from build123d import *

# Parameters (mm, degrees)
EXTRUDE_1_DEPTH     = 12
SKETCH_4_W          = 56
SKETCH_4_H          = 3
SKETCH_4_H_2        = 1
EXTRUDE_2_DEPTH     = 12
SKETCH_5_R          = 1.15
SKETCH_5_R_2        = 2.6
CUT_EXTRUDE_2_DEPTH = 53.211370172
SKETCH_7_R          = 1
CUT_EXTRUDE_3_DEPTH = 10


with BuildPart() as part:
    # 草图2 → 凸台-拉伸1 (new body)
    with BuildSketch(Plane(origin=(0, 0, 0), x_dir=(1, 0, 0), z_dir=(0, 1, 0))):
        Polygon((-10.725663717, 9.92920354), (45.274336283, 9.92920354), (45.274336283, -22.07079646), (-10.725663717, -22.07079646), (-10.725663717, -7.07079646), (-10.725663717, 1.92920354), align=None)
        Polygon((-9.725663717, -7.07079646), (-9.725663717, -14.07079646), (44.274336283, -14.07079646), (44.274336283, 8.92920354), (-9.725663717, 8.92920354), (-9.725663717, 0.92920354), align=None, mode=Mode.SUBTRACT)
    extrude(amount=EXTRUDE_1_DEPTH)

    # 草图4 → 凸台-拉伸2 (add)
    with BuildSketch(Plane(origin=(0, 0, 0), x_dir=(1, 0, 0), z_dir=(0, 1, 0))):
        with Locations((17.274336283, 11.42920354)):
            Rectangle(SKETCH_4_W, SKETCH_4_H)
        with Locations((17.274336283, -22.57079646)):
            Rectangle(SKETCH_4_W, SKETCH_4_H_2)
    extrude(amount=EXTRUDE_2_DEPTH)

    # 草图5 → 切除-拉伸2 (cut, through all)
    with BuildSketch(Plane(origin=(0, 12, 0), x_dir=(1, 0, 0), z_dir=(0, 1, 0))):
        with Locations(Location((-5.725663717, 10.92920354, 0), (0, 0, 270))):
            Circle(SKETCH_5_R)
        with Locations(Location((40.274336283, 10.92920354, 0), (0, 0, 270))):
            Circle(SKETCH_5_R)
        with Locations(Location((-5.725663717, -18.57079646, 0), (0, 0, 270))):
            Circle(SKETCH_5_R_2)
        with Locations(Location((40.274336283, -18.57079646, 0), (0, 0, 270))):
            Circle(SKETCH_5_R_2)
    extrude(amount=-CUT_EXTRUDE_2_DEPTH, mode=Mode.SUBTRACT)

    # 草图7 → 切除-拉伸3 (cut)
    with BuildSketch(Plane(origin=(0, 12, 0), x_dir=(1, 0, 0), z_dir=(0, 1, 0))):
        with Locations(Location((17.274336283, -19.142973174, 0), (0, 0, 270))):
            Circle(SKETCH_7_R)
    extrude(amount=-CUT_EXTRUDE_3_DEPTH, mode=Mode.SUBTRACT)


solid = part.part
Can you work these out from the model? Positions are in its coordinate system, mm. A direction names the side the tool comes from. Give positions to 0.01 mm unless a question says otherwise; leave off trailing zeros. Order: outer loops, then holes, each group sorted by start corner. A loop starts at its lowest first (then second) coordinate and runs counter-clockwise, first axis right, second up. Notation, with made-up numbers: (78, 83) - (115, 83) arc R13 ccw to (115, 94) - close; hole circle Ø9 at (19, 55.5). An arc over 180 degrees is marked (long way). Write each question's results on one line, items separated by ' | '.
1) If we mould it in two halves opening along X, with no side actions, what happens to faces 4 (the face through (45.274, 6, 5)), 5 (the face through (15.1, 12, 14.3)), 6 (the face through (-10.726, 6, 5)), 7 (the face through (-5.38, 6.084, -9.832))? For each: pulls with the +X half, pulls with the -X half, needs draft (parallel to the pull), parting line crosses it, or undercut.
Final values:
face 4: pulls with the +X half | face 5: needs draft | face 6: pulls with the -X half | face 7: undercut
2) I'm going to push a flat-ended pin straight in: pin 1 Ø1.6 at (x, z) = (17.27, 19.14) entering from +Y. Where does the tip first touch, or does it pass through?
Final values:
pin 1: stops at y = 2
3) Suppose I cut it at C-C, the plane y = 5.25. Write out the boundary of the cut face in (x, z).
Final values:
outline: (-10.73, -12.93) - (45.27, -12.93) - (45.27, 23.07) - (-10.73, 23.07) - close; hole (-9.73, -8.93) - (44.27, -8.93) - (44.27, 14.07) - (-9.73, 14.07) - close; hole circle Ø5.2 at (-5.73, 18.57); hole circle Ø2.3 at (-5.73, -10.93); hole circle Ø2 at (17.27, 19.14); hole circle Ø5.2 at (40.27, 18.57); hole circle Ø2.3 at (40.27, -10.93)
4) On a 3-axis mill with a long thin cutter (end or side, diameter ignored), from which of +Z, -Z, +X, -X, +Y, -Y can I reach the whole of each face in a straight line? I mean faces 1 (the face through (13, 0, 14.3)), 2 (the face through (17.95, 7.07, 18.406)), 3 (the face through (17, 6, 14.071)). Say none if no direction works.
Final values:
face 1: +Z, -Z, +X, -X, -Y | face 2: +Y | face 3: +Y, -Y
5) Suppose I cut it at A-A, the plane x = 13. Write out the boundary of the cut face in (y, z).
Final values:
outline: (0, -12.93) - (12, -12.93) - (12, -8.93) - (0, -8.93) - close; (0, 14.07) - (12, 14.07) - (12, 23.07) - (0, 23.07) - close
6) Please list where these lines run through material, in increasing order: line 1 along Z through (x, y) = (13, 2.25); line 2 along X through (y, z) = (7, 2.5); line 3 along X through (y, z) = (5, -10.5). Write a range as [from, to].
Final values:
line 1: z = [-12.93, -8.93], [14.07, 23.07] | line 2: x = [-10.73, -9.73], [44.27, 45.27] | line 3: x = [-10.73, -6.79], [-4.66, 39.21], [41.34, 45.27]
7) Suppose I cut it at B-B, the plane z = 0. Write out the boundary of the cut face in (x, y), then the cut area to 3 significant figures.
Final values:
outline: (-10.73, 0) - (-9.73, 0) - (-9.73, 12) - (-10.73, 12) - close; (44.27, 0) - (45.27, 0) - (45.27, 12) - (44.27, 12) - close | area: 24.0 mm^2
